```python
from build123d import *

# Parameters (mm, degrees)
SKETCH1_W               = 47.86122
SKETCH1_H               = 73.00722
SKETCH1_R               = 2.5527
BOSS_EXTRUDE1_DEPTH     = 22.14118
CUT_EXTRUDE1_DEPTH      = 49.943022892
CUT_EXTRUDE1_DEPTH_BACK = 49.943022892
CHAMFER1_SIZE           = 2.54
CUT_EXTRUDE2_DEPTH      = 49.943022892
SKETCH5_W               = 43.18
SKETCH5_H               = 22.86
CUT_EXTRUDE3_DEPTH      = 0.254
SKETCH7_R               = 2.54
BOSS_EXTRUDE3_DEPTH     = 20.32
FILLET1_R               = 2.54
FILLET2_R               = 1.27


with BuildPart() as part:
    # Sketch1 → Boss-Extrude1 (new body)
    with BuildSketch(Plane(origin=(0, 0, 0), x_dir=(1, 0, 0), z_dir=(0, 1, 0))):
        Rectangle(SKETCH1_W, SKETCH1_H)
        with Locations(Location((-19.14525, 31.90875, 0), (0, 0, 270))):
            Circle(SKETCH1_R, mode=Mode.SUBTRACT)
        with Locations(Location((19.14525, 31.90875, 0), (0, 0, 270))):
            Circle(SKETCH1_R, mode=Mode.SUBTRACT)
        with Locations(Location((19.14525, -31.90875, 0), (0, 0, 270))):
            Circle(SKETCH1_R, mode=Mode.SUBTRACT)
        with Locations(Location((-19.14525, -31.90875, 0), (0, 0, 270))):
            Circle(SKETCH1_R, mode=Mode.SUBTRACT)
    extrude(amount=BOSS_EXTRUDE1_DEPTH)

    # Sketch2 → Cut-Extrude1 (cut, two sides: drawn at the far end of the back side and taken through both)
    with BuildSketch(Plane(origin=(0, 0, 0), x_dir=(0, 0, -1), z_dir=(1, 0, 0)).offset(-CUT_EXTRUDE1_DEPTH_BACK)):
        Polygon((14.7066, 22.14118), (-14.7066, 22.14118), (-27.259853255, 10.83818), (-36.50361, 10.83818), (-45.550551374, 42.074053009), (0, 43.630244296), (45.550551374, 42.074053009), (36.50361, 10.83818), (27.259853255, 10.83818), align=None)
    extrude(amount=CUT_EXTRUDE1_DEPTH + CUT_EXTRUDE1_DEPTH_BACK, mode=Mode.SUBTRACT)

    # Chamfer1
    chamfer1_edges = [part.edges().sort_by_distance(p)[0] for p in [
        (-23.93061, 5.41909, -36.50361),
        (23.93061, 5.41909, -36.50361),
        (23.93061, 5.41909, 36.50361),
        (-23.93061, 5.41909, 36.50361),
    ]]
    chamfer(chamfer1_edges, length=CHAMFER1_SIZE)

    # Sketch4 → Cut-Extrude2 (cut, through all)
    with BuildSketch(Plane(origin=(0, 0, 0), x_dir=(1, 0, 0), z_dir=(0, 1, 0))):
        Polygon((-12.7, 36.50361), (-7.62, 31.93161), (7.62, 31.93161), (12.7, 36.50361), align=None)
        Polygon((-12.7, -36.50361), (-7.62, -31.93161), (7.62, -31.93161), (12.7, -36.50361), align=None)
    extrude(amount=CUT_EXTRUDE2_DEPTH, mode=Mode.SUBTRACT)

    # Sketch5 → Cut-Extrude3 (cut)
    with BuildSketch(Plane(origin=(0, 22.14118, 0), x_dir=(1, 0, 0), z_dir=(0, 1, 0))):
        Rectangle(SKETCH5_W, SKETCH5_H)
    extrude(amount=-CUT_EXTRUDE3_DEPTH, mode=Mode.SUBTRACT)

    # Sketch7 → Boss-Extrude3 (add)
    with BuildSketch(Plane(origin=(0, 0, 0), x_dir=(1, 0, 0), z_dir=(0, 1, 0))):
        with Locations(Location((-19.14525, 20.47875, 0), (0, 0, 90))):
            Circle(SKETCH7_R)
    extrude(amount=BOSS_EXTRUDE3_DEPTH)

    # Fillet1
    # the kernel refuses this fillet: 2.54 mm, written as the material it takes off along each edge
    with BuildSketch(Plane(origin=(-19.14525, 20.32, -20.47875), x_dir=(0, 0, -1), z_dir=(1, 0, 0))) as fillet1_piece_1_section:
        with BuildLine():
            CenterArc((2.54 - FILLET1_R, -FILLET1_R), FILLET1_R, 0, 90)
            Line((2.54 - FILLET1_R, 0), (2.54, 0))
            Line((2.54, 0), (2.54, -FILLET1_R))
        make_face()
    fillet1_piece_1 = revolve(axis=Axis((-19.14525, 20.32, -20.47875), (0, 1, 0)), mode=Mode.PRIVATE)
    fillet1_piece_1 = split(fillet1_piece_1, bisect_by=Plane(origin=(-19.14525, 19.033531864, -18.157992912), z_dir=(0, 0.7431448254773929, -0.6691306063588597)), keep=Keep.TOP, mode=Mode.PRIVATE)
    add(fillet1_piece_1, mode=Mode.SUBTRACT)

    # Fillet2
    fillet2_edges = [part.edges().sort_by_distance(p)[0] for p in [
        (-12.7, 5.41909, 36.50361),
        (12.7, 5.41909, 36.50361),
        (7.62, 5.41909, 31.93161),
        (-7.62, 5.41909, 31.93161),
        (-23.93061, 5.41909, 33.96361),
        (-23.93061, 5.41909, -33.96361),
        (21.39061, 5.41909, -36.50361),
        (-21.39061, 5.41909, -36.50361),
        (23.93061, 5.41909, 33.96361),
        (23.93061, 5.41909, -33.96361),
        (21.39061, 5.41909, 36.50361),
        (-21.39061, 5.41909, 36.50361),
        (12.7, 5.41909, -36.50361),
        (-12.7, 5.41909, -36.50361),
        (-7.62, 5.41909, -31.93161),
        (7.62, 5.41909, -31.93161),
    ]]
    fillet(fillet2_edges, radius=FILLET2_R)


solid = part.part
```
Verification items for the finished model (mm, model axes). A direction names the side the tool comes from. Coordinates: 2 decimals unless noted, no trailing zeros. Loops run counter-clockwise (first coordinate to the right, second up) from the corner with the lowest first, then second, coordinate; pieces in that order, holes last. Notation, with made-up numbers: (46.5, 1.5) -> (73.5, 1.5) arc R20 ccw to (73.5, 11.5) -> close; hole circle Ø11 at (59.25, 40). An arc over 180 degrees is marked (long way). Answer in a Markdown table with one row per item. Add a question column.
1. Access from +Z, -Z, +X, -X, +Y, -Y to the whole of each face (thin tool, end or side, straight path). Record for faces 4 (the face through (0, 10.838, 31)), 5 (the face through (0, 21.887, 0)), 6 (the face through (-10.19, 5.343, 34.245)), 7 (the face through (0, 5, -31.932)).
2. Section check A-A, the plane x = 15. Enter the section's corners in (y, z), then the cut area to 3 significant figures.
3. Section check D-D, the plane z = 26. Enter the section's corners in (x, y).
4. Material ranges on probe 1 along Z at (x, y) = (-19, 4.25); probe 2 along Z at (x, y) = (-17.5, 8.5); probe 3 along Y at (x, z) = (-11.5, -8), recorded low to high. Write a range as [from, to].
5. Section check B-B, the plane x = -2. Enter the section's corners in (y, z), then the cut area to 3 significant figures.
6. Depth check by flat-ended pin: P1, Ø3, axis at x = 9, z = 32, coming from the +Y side; P2, Ø8.5, axis at x = 3, y = 6.5, coming from the +Z side; P3, Ø4, axis at x = -7.5, y = 13, coming from the +Z side. Enter the tip coordinate at first touch or a pass-through.
7. Section check C-C, the plane y = 6.75. Give the number of separate pieces and of enclosed holes in the cut face, then the cut area to 3 significant figures.
8. Draft check along Z on faces 1 (the face through (-22.648, 5.343, 35.246)), 2 (the face through (17, 5, -36.504)), 3 (the face through (18.17, 5.34, -29.55)). Enter one of: +Z half, -Z half, draft (parallel to the pull), parting line (faces both ways), or undercut.
Derived:
| question | item | result |
|---|---|---|
| 1 | face 4 | +Z, +X, -X, +Y |
| 1 | face 5 | +Y |
| 1 | face 6 | +Z, +Y, -Y |
| 1 | face 7 | -Z, +Y, -Y |
| 2 | outline | (0, -36.5) -> (10.84, -36.5) -> (10.84, -27.26) -> (22.14, -14.71) -> (22.14, -11.43) -> (21.89, -11.43) -> (21.89, 11.43) -> (22.14, 11.43) -> (22.14, 14.71) -> (10.84, 27.26) -> (10.84, 36.5) -> (0, 36.5) -> close |
| 2 | area | 1,260 mm² |
| 3 | outline | (-23.93, 0) -> (23.93, 0) -> (23.93, 11.97) -> (-23.93, 11.97) -> close |
| 4 | probe 1 | z = [-36.5, -34.46], [-29.36, 29.36], [34.46, 36.5] |
| 4 | probe 2 | z = [-36.5, -33.86], [-29.96, 29.96], [33.86, 36.5] |
| 4 | probe 3 | y = [0, 21.89] |
| 5 | outline | (0, -31.93) -> (10.84, -31.93) -> (10.84, -27.26) -> (22.14, -14.71) -> (22.14, -11.43) -> (21.89, -11.43) -> (21.89, 11.43) -> (22.14, 11.43) -> (22.14, 14.71) -> (10.84, 27.26) -> (10.84, 31.93) -> (0, 31.93) -> close |
| 5 | area | 1,160 mm² |
| 6 | P1 | stops at y = 10.84 |
| 6 | P2 | stops at z = 31.94 |
| 6 | P3 | stops at z = 27.08 |
| 7 | separate pieces | 1 |
| 7 | enclosed holes | 4 |
| 7 | area | 3,210 mm² |
| 8 | face 1 | +Z half |
| 8 | face 2 | -Z half |
| 8 | face 3 | undercut |
